Answer from the drawing. Dimensions are ordinates in mm from the lowest x, y and z of the part. A direction names the side the tool comes from. Give positions to 0.01 mm unless a question says otherwise; leave off trailing zeros. Write each loop counter-clockwise with the first axis right and the second up, starting at its lowest first coordinate (ties: lowest second). Pieces come first, ordered by that corner, then holes. Notation, with made-up numbers: (-8.75, 71) -> (41.25, 71) arc R13 cw to (41.25, 79) -> close; hole circle Ø5 at (-30.5, -2.5). An arc over 180 degrees is marked (long way). Put each result on its own line as item: value. Start each with the question number.
1) For the marked faces 5, 6, 7 and 8, determine the directions among +Z, -Z, +X, -X, +Y, -Y from which every point of the face is accessible in a straight line to the end or side of a thin tool.
2) A cutting plane is placed at D-D (z = 20). Write down the section's boundary in (x, y).
3) A cutting plane is placed at A-A (x = 4). Write down the section's boundary in (y, z).
4) A cutting plane is placed at C-C (z = 17.75). Write down the section's boundary in (x, y) (1 decimal).
5) Find the intervals of material crossed by line 1 along Y through (x, z) = (35, 2.2); line 2 along Y through (x, z) = (17, 14.25); line 3 along X through (y, z) = (2, 17), in increasing order. Write a range as from..to.
6) Flat-ended cylindrical pins translate along their axes: pin 1 Ø4.5 at (y, z) = (27.5, 9.5) entering from -X; pin 2 Ø6 at (y, z) = (26, 10) entering from +X; pin 3 Ø1 at (x, y) = (22.5, 16) entering from +Z; pin 4 Ø2 at (x, z) = (23.5, 8) entering from +Y. Find the tip coordinate at first contact, or state that the pin passes through.
7) For a pull along Y with two mould halves and no side action, classify the marked faces 1, 2, 3 and 4 as released by +Y, released by -Y, zero draft, split by the parting line, or undercut.
8) A cutting plane is placed at B-B (y = 26.5). Write down the section's boundary in (x, z).
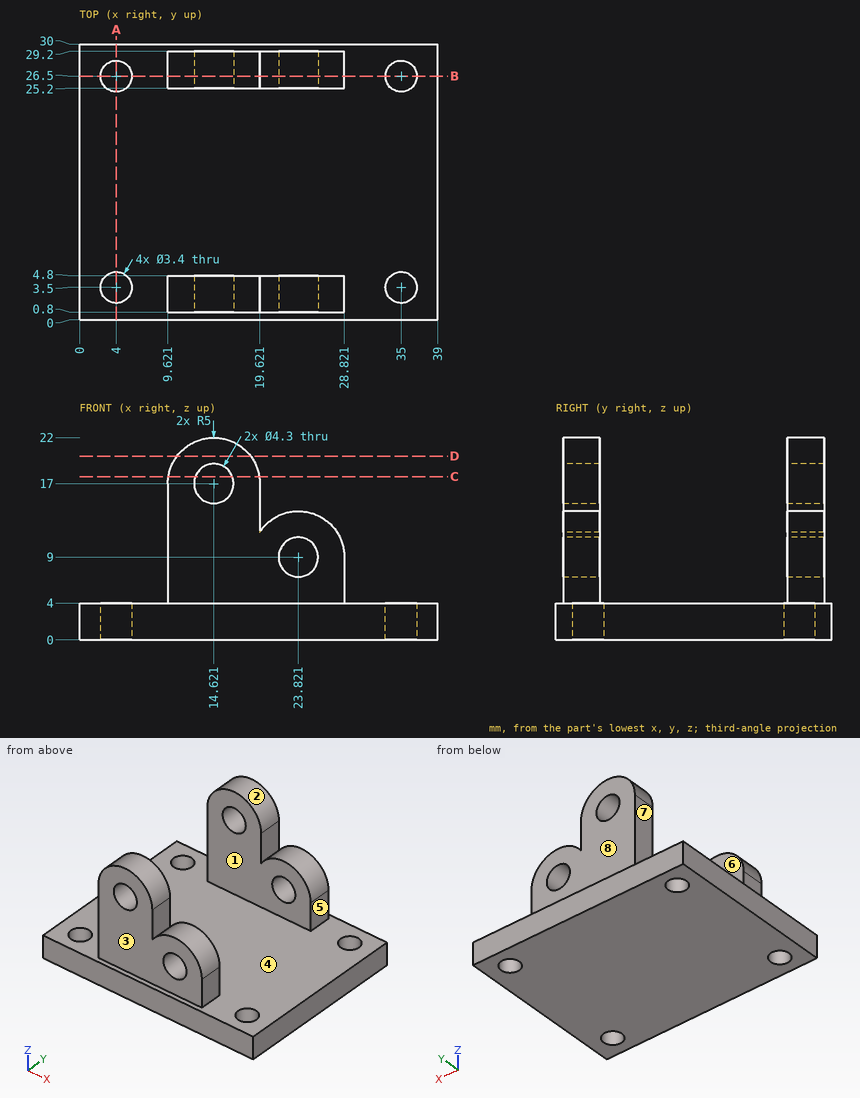
Reply:
1. face 5: +Z, +X, +Y, -Y
1. face 6: +Z, +X, -X
1. face 7: +Z, -X, +Y, -Y
1. face 8: +Z, +X, -X, +Y
2. outline: (10.62, 0.8) -> (18.62, 0.8) -> (18.62, 4.8) -> (10.62, 4.8) -> close; (10.62, 25.2) -> (18.62, 25.2) -> (18.62, 29.2) -> (10.62, 29.2) -> close
3. outline: (0, 0) -> (1.8, 0) -> (1.8, 4) -> (0, 4) -> close; (5.2, 0) -> (24.8, 0) -> (24.8, 4) -> (5.2, 4) -> close; (28.2, 0) -> (30, 0) -> (30, 4) -> (28.2, 4) -> close
4. outline: (9.7, 0.8) -> (12.6, 0.8) -> (12.6, 4.8) -> (9.7, 4.8) -> close; (9.7, 25.2) -> (12.6, 25.2) -> (12.6, 29.2) -> (9.7, 29.2) -> close; (16.6, 0.8) -> (19.6, 0.8) -> (19.6, 4.8) -> (16.6, 4.8) -> close; (16.6, 25.2) -> (19.6, 25.2) -> (19.6, 29.2) -> (16.6, 29.2) -> close
5. line 1: y = 0..1.8, 5.2..24.8, 28.2..30
5. line 2: y = 0.8..4.8, 25.2..29.2
5. line 3: x = 9.62..12.47, 16.77..19.62
6. pin 1: stops at x = 9.62
6. pin 2: stops at x = 28.82
6. pin 3: stops at z = 4
6. pin 4: passes through
7. face 1: undercut
7. face 2: zero draft
7. face 3: released by -Y
7. face 4: undercut
8. outline: (0, 0) -> (2.3, 0) -> (2.3, 4) -> (0, 4) -> close; (5.7, 0) -> (33.3, 0) -> (33.3, 4) -> (28.82, 4) -> (28.82, 9) arc R5 ccw to (19.62, 11.71) -> (19.62, 17) arc R5 ccw to (9.62, 17) -> (9.62, 4) -> (5.7, 4) -> close; (36.7, 0) -> (39, 0) -> (39, 4) -> (36.7, 4) -> close; hole circle Ø4.3 at (14.62, 17); hole circle Ø4.3 at (23.82, 9)
